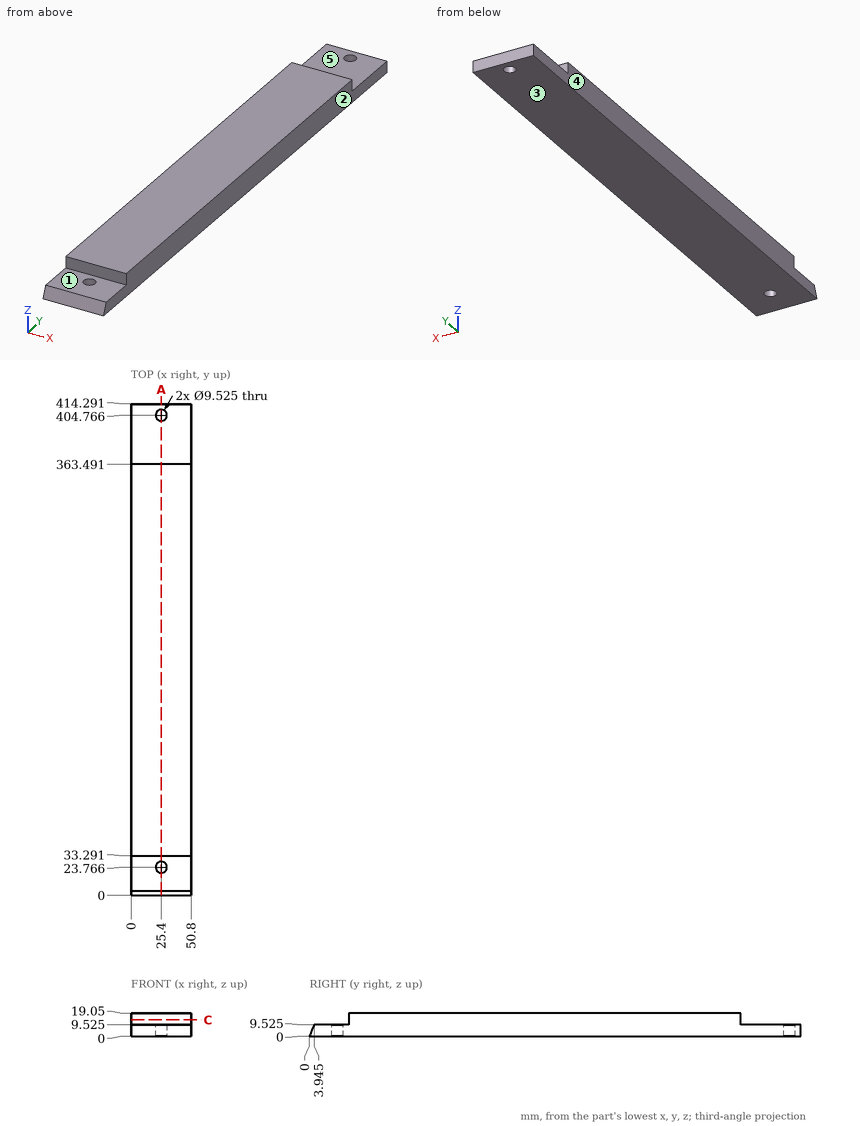
Source: three-view drawing plus pictorial views. Frame: mm from the lowest corner of the part. A direction names the side the tool comes from. Round coordinates to 2 decimals unless told otherwise and drop trailing zeros. Loops run counter-clockwise (first coordinate to the right, second up) from the corner with the lowest first, then second, coordinate; pieces in that order, holes last.
Q1. Access query for the marked faces 4 and 5. Directions: +Z, -Z, +X, -X, +Y, -Y. A direction counts if a zero-diameter tool reaches every point of the face in a straight line with its end or side. Return the directions, or none.
Q2. Ray query, line 1 (Y direction, x = 25.4, z = 5.5); line 2 (Y direction, x = 25.4, z = 2.5) (1 decimal); line 3 (Y direction, x = 5, z = 14). Return the intervals inside material, ascending.
Q3. First-contact query: P1, Ø4, axis at x = 16.5, z = 17, coming from the -Y side; P2, Ø8, axis at x = 30, z = 7.5, coming from the -Y side; P3, Ø4, axis at x = 12, z = 10.5, coming from the -Y side; P4, Ø7.5, axis at x = 25.4, y = 404.77, coming from the -Z side. Flat tips, straight axial feed; report the tip coordinate or a pass-through.
Q4. Section A-A, the plane x = 25.4. State how many separate pieces and enclosed holes the cut face has, plus the area to 3 significant figures.
Q5. Mould query, pull axis Z, two halves, no side actions, for the marked faces 1, 2 and 3. Classes: pulls with the +Z half, pulls with the -Z half, needs draft (parallel to the pull), parting line crosses it, or undercut.
Q6. Section C-C, the plane z = 13.5. Return loops of the section in (x, y), plus the area to 3 significant figures.
Solutions:
1. face 4: +Z, -Z, -X, +Y, -Y
1. face 5: +Z, +X, -X, +Y
2. line 1: y = 2.28 to 19, 28.53 to 400, 409.53 to 414.29
2. line 2: y = 1 to 19, 28.5 to 400, 409.5 to 414.3
2. line 3: y = 33.29 to 363.49
3. P1: stops at y = 33.29
3. P2: stops at y = 1.45
3. P3: stops at y = 3.52
3. P4: passes through
4. separate pieces: 3
4. enclosed holes: 0
4. area: 6,890 mm2
5. face 1: pulls with the +Z half
5. face 2: needs draft
5. face 3: pulls with the -Z half
6. outline: (0, 33.29) - (50.8, 33.29) - (50.8, 363.49) - (0, 363.49) - close
6. area: 16,800 mm2
